CAD build for the part. Positions are in the model's coordinates, mm. A direction names the side the tool comes from. Round coordinates to 2 decimals unless told otherwise and drop trailing zeros. Order: outer loops, then holes, each group sorted by start corner. A loop starts at its lowest first (then second) coordinate and runs counter-clockwise, first axis right, second up. Notation, with made-up numbers: (48.5, 20.25) -> (55.5, 20.25) arc R8 cw to (55.5, 33.25) -> close; hole circle Ø8 at (72, 84). An arc over 180 degrees is marked (long way). Return JSON: item names as keys, results as strings. Group by question number.
Q1. Cut at B-B (y = 8.45). Write the cut outline in (x, z), then the cut area to 3 significant figures.
Q2. Cut at C-C (z = 2.9). Write the cut outline in (x, y), then the cut area to 3 significant figures.
Q3. Cut at D-D (x = 11). Write the cut outline in (y, z), then the cut area to 3 significant figures.
Q4. Flat gauge pin, fed straight in: pin 1 (1 mm diameter, centred on y = 15, z = 3, fed in from -X). Where does the tip first touch, or does it go through?
Q5. Cut at A-A (y = 4.5). Write the cut outline in (x, z).
Q6. Which spindle directions (+Z, -Z, +X, -X, +Y, -Y) get a long thin tool onto all of the face, cutting with end or side? Do faces 4 (the flat face through (0, 6, 2)), 5 (the flat face through (-18, 7, 2)). Say none if no direction does.
Q7. Probe line 1 along X through (y, z) = (8.75, 2.8); line 2 along X through (y, z) = (12.5, 2.8); line 3 along X through (y, z) = (10.5, 3.4). List the from-to ranges inside material, lowest first.
Q8. Mould opens along X. For faces 1 (the flat face through (23, 6, 2)), 2 (the flat face through (27, 0, 2)), 3 (the flat face through (31.5, 7, 2)) say: +X half, -X half, draft (parallel to the pull), parting line (faces both ways), or undercut.
from build123d import *

# Parameters (mm, degrees)
BOSS_EXTRUDE1_DEPTH = 4
SKETCH2_R           = 1.0668
SKETCH2_R_2         = 2.9
CUT_EXTRUDE1_DEPTH  = 4


with BuildPart() as part:
    # Sketch1 → Boss-Extrude1 (new body)
    with BuildSketch(Plane.XY):
        with BuildLine():
            Line((-18, 0), (0, 0))
            Line((0, 0), (0, 12.58))
            Line((0, 12.58), (23, 12.58))
            Line((23, 12.58), (23, 0))
            Line((23, 0), (31.5, 0))
            Line((31.5, 0), (31.5, 14))
            ThreePointArc((31.5, 14), (30.328427125, 16.828427125), (27.5, 18))
            Line((27.5, 18), (-14, 18))
            ThreePointArc((-14, 18), (-16.828427125, 16.828427125), (-18, 14))
            Line((-18, 14), (-18, 0))
        make_face()
    extrude(amount=BOSS_EXTRUDE1_DEPTH)

    # Sketch2 → Cut-Extrude1 (cut)
    with BuildSketch(Plane.XY.offset(4)):
        with Locations((25.1968, 6.3119)):
            Circle(SKETCH2_R)
        with Locations((-2.3368, 6.3119)):
            Circle(SKETCH2_R)
        with Locations((-11.476, 8.45)):
            Circle(SKETCH2_R_2)
    extrude(amount=-CUT_EXTRUDE1_DEPTH, mode=Mode.SUBTRACT)


solid = part.part
Solution:
{
 "1": {"outline": "(-18, 0) -> (-14.38, 0) -> (-14.38, 4) -> (-18, 4) -> close; (-8.58, 0) -> (0, 0) -> (0, 4) -> (-8.58, 4) -> close; (23, 0) -> (31.5, 0) -> (31.5, 4) -> (23, 4) -> close", "area": "82.8 mm²"},
 "2": {"outline": "(-18, 0) -> (0, 0) -> (0, 12.58) -> (23, 12.58) -> (23, 0) -> (31.5, 0) -> (31.5, 14) arc R4 ccw to (27.5, 18) -> (-14, 18) arc R4 ccw to (-18, 14) -> close; hole circle Ø5.8 at (-11.48, 8.45); hole circle Ø2.13 at (-2.34, 6.31); hole circle Ø2.13 at (25.2, 6.31)", "area": "561 mm²"},
 "3": {"outline": "(12.58, 0) -> (18, 0) -> (18, 4) -> (12.58, 4) -> close", "area": "21.7 mm²"},
 "4": {"pin 1": "stops at x = -17.97"},
 "5": {"outline": "(-18, 0) -> (0, 0) -> (0, 4) -> (-18, 4) -> close; (23, 0) -> (31.5, 0) -> (31.5, 4) -> (23, 4) -> close"},
 "6": {"face 4": "+Z, -Z, -Y", "face 5": "+Z, -Z, -X, +Y, -Y"},
 "7": {"line 1": "x = -18 to -14.36, -8.59 to 0, 23 to 31.5", "line 2": "x = -18 to 0, 23 to 31.5", "line 3": "x = -18 to -13.53, -9.42 to 0, 23 to 31.5"},
 "8": {"face 1": "undercut", "face 2": "draft", "face 3": "+X half"}
}
